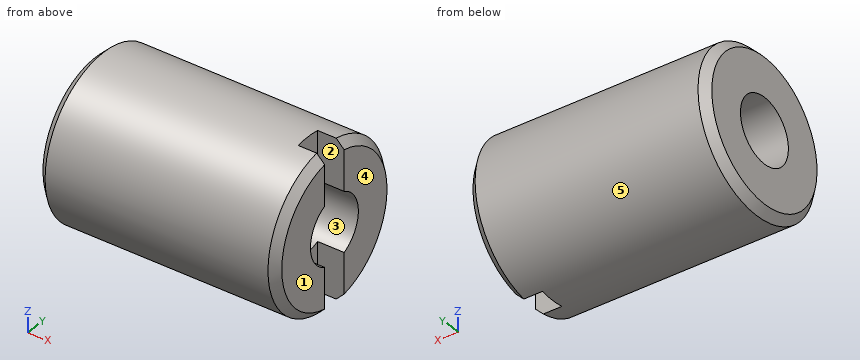
Autodesk Inventor part; units mm, degrees
ref_plane "YZ Plane" through (0, 0, 0) normal (1, 0, 0) x (0, 1, 0)
ref_plane "XZ Plane" through (0, 0, 0) normal (0, 1, 0) x (-1, 0, 0)
ref_plane "XY Plane" through (0, 0, 0) normal (0, 0, 1) x (1, 0, 0)
sketch "スケッチ1" plane through (0, 0, 0) normal (0, 1, 0) x (-1, 0, 0)
  line L0 (0, 0) -> (9, 0)
  line L1 (9, 0) -> (9, -3)
  line L2 (9, -3) -> (0, -3)
  line L3 (0, -3) -> (0, 0)
  dimension "d0" = 9
  dimension "d1" = 3
revolve "回転1" add sketch "スケッチ1" angle 360 about axis through (0, 0, 0) along (-1, 0, 0)
sketch "スケッチ2" plane through (0, 0, 0) normal (1, 0, 0) x (0, 0, -1)
  point P0 (0, 0)
  point P1 (0, 0)
hole "穴1" at (0, 0, 0) direction (-1, 0, 0) diameter 2.459 end through all
sketch "スケッチ3" plane through (0, 0, 0) normal (1, 0, 0) x (0, 0, -1)
  circle A0 centre (0, 0) radius 3
  line L0 (3, 0) -> (-3, 0)
  line L1 (3, -0.5) -> (-3, -0.5)
  line L2 (3, 0.5) -> (-3, 0.5)
  line L3 (3, 0.5) -> (3, -0.5)
  line L4 (-3, 0.5) -> (-3, -0.5)
  point P0 (-2.958, -0.5)
  point P1 (2.958, -0.5)
  point P2 (2.958, 0.5)
  point P3 (-2.958, 0.5)
  dimension "d10" = 0.5
extrude "押し出し1" cut sketch "スケッチ3" against normal blind 1 contours L0 A0 L2 | A0 L1 L0
chamfer "面取り1" distance 0.3 angle 45 3 edges at (-9, 0, 3) (0, 3, 0) (0, -3, 0)
properties part number "ARU-309S" material "ステンレス鋼 AISI 304"
Could you check a few things on this model? Use its own coordinates, in mm. Face numbers are marked on the shaded views. A direction names the side the tool comes from. Round coordinates to 2 decimals unless told otherwise and drop trailing zeros. Loops run counter-clockwise (first coordinate to the right, second up) from the corner with the lowest first, then second, coordinate; pieces in that order, holes last. Notation, with made-up numbers: (9.5, 16) - (33.5, 16) arc R13 cw to (33.5, 22) - close; hole circle Ø6 at (-17, -25). An arc over 180 degrees is marked (long way). Write item = value, one per line.
1) Imagine slicing it at C-C (x = -6.75). Please give me the cut outline in (y, z).
Computed:
outline = circle Ø6 at (0, 0); hole circle Ø2.46 at (0, 0)
2) Imagine slicing it at A-A (z = 0). Please give me the cut outline in (x, y), and give its area (3 significant figures).
Computed:
outline = (-9, -2.7) - (-8.7, -3) - (-0.3, -3) - (0, -2.7) - (0, -1.23) - (-9, -1.23) - close; (-9, 1.23) - (0, 1.23) - (0, 2.7) - (-0.3, 3) - (-8.7, 3) - (-9, 2.7) - close
area = 31.7 mm2
3) I'm going to push flat-ended pins straight in: P1, Ø0.5, axis at x = -0.5, z = -2.5, coming from the -Y side; P2, Ø0.5, axis at x = -0.5, z = 2, coming from the +Y side; P3, Ø1.1, axis at x = -0.5, z = -2, coming from the +Y side. Where does each tip first touch, or does it pass through?
Computed:
P1 = -1.98
P2 = 2.44
P3 = 2.63
4) On a 3-axis mill with a long thin cutter (end or side, diameter ignored), from which of +Z, -Z, +X, -X, +Y, -Y can I reach the whole of each face in a straight line? I mean the marked faces 1 and 2. Say none if no direction works.
Computed:
face_1 = +Z, -Z, +X, +Y, -Y
face_2 = +Z, -Z, +X
5) Imagine slicing it at B-B (y = 0). Please give me the cut outline in (x, z), and give its area (3 significant figures).
Computed:
outline = (-9, -2.7) - (-8.7, -3) - (-1, -3) - (-1, -1.23) - (-9, -1.23) - close; (-9, 1.23) - (-1, 1.23) - (-1, 3) - (-8.7, 3) - (-9, 2.7) - close
area = 28.2 mm2
6) I need wall thicknesses on line 1 along Y through (x, z) = (-6, 0); line 2 along Z through (x, y) = (-6.5, 0.5). Which ranges of each line are inside material? Lowest first, please. Write a range as from..to.
Computed:
line_1 = -3..-1.23, 1.23..3
line_2 = -2.96..-1.12, 1.12..2.96
7) If we mould it in two halves opening along Z, with no side actions, what happens to the marked faces 3, 4 and 5? For each: pulls with the +Z half, pulls with the -Z half, needs draft (parallel to the pull), parting line crosses it, or undercut.
Computed:
face_3 = undercut
face_4 = needs draft
face_5 = parting line crosses it
